Verification items for this drawing (mm, ordinates from the low corner). Give positions to 0.01 mm unless a question says otherwise; leave off trailing zeros. Write each loop counter-clockwise with the first axis right and the second up, starting at its lowest first coordinate (ties: lowest second). Pieces come first, ordered by that corner, then holes. Notation, with made-up numbers: (25, -39) -> (66, -39) arc R26 cw to (66, -20) -> close; hole circle Ø9 at (-7.5, 60). An arc over 180 degrees is marked (long way). Answer as a JSON object with one key per item and string values.
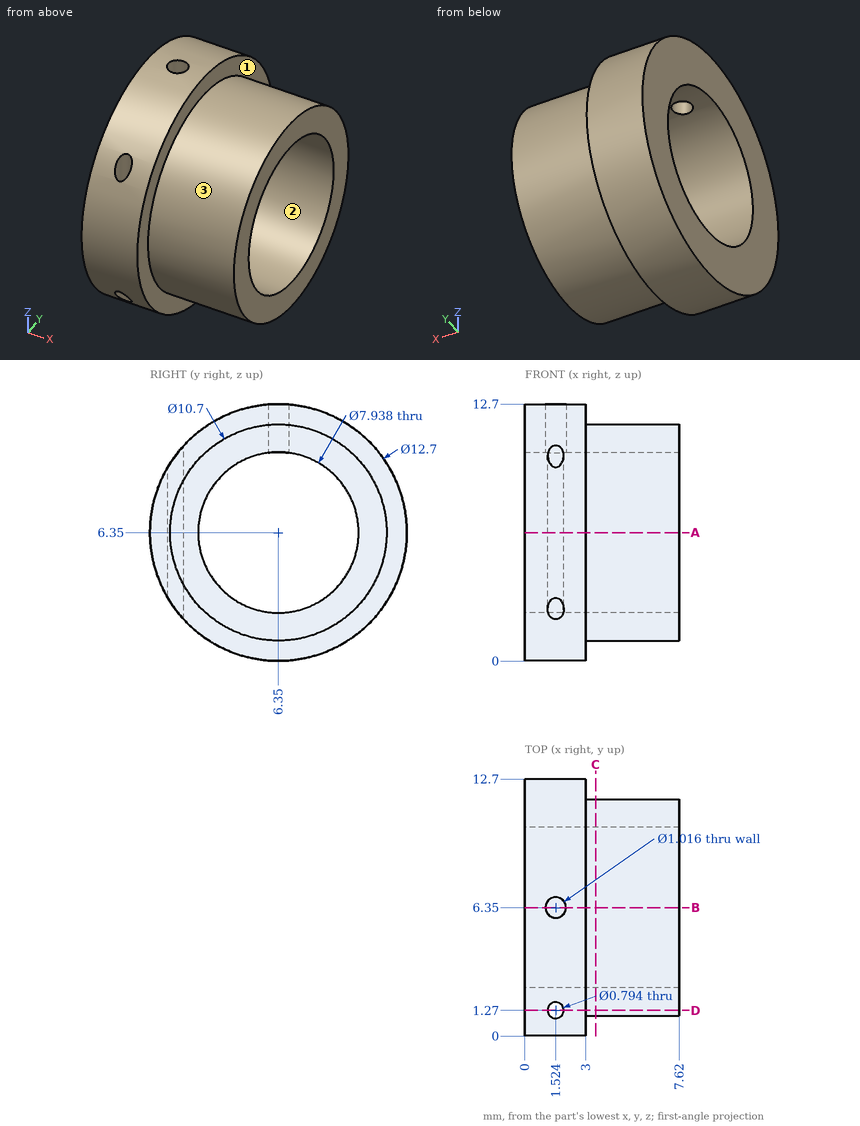
1. Scan lines: L1, parallel to Y at x = 1.5, z = 9 (1 decimal); L2, parallel to Z at x = 6.25, y = 6.5 (1 decimal); L3, parallel to Z at x = 1.75, y = 5.5. Record each from-to range of solid material in increasing order. Write a range as [from, to].
Determined:
{"L1": "[0.6, 0.9], [1.7, 3.4], [9.3, 12.1]", "L2": "[1, 2.4], [10.3, 11.7]", "L3": "[0.06, 2.47], [10.23, 12.64]"}
2. Sectioned sample at D-D, the plane y = 1.27. Enter the section's corners in (x, z).
Determined:
{"outline": "(0, 2.54) -> (1.13, 2.54) -> (1.13, 10.16) -> (0, 10.16) -> close; (1.92, 2.54) -> (3, 2.54) -> (3, 4.67) -> (7.62, 4.67) -> (7.62, 8.03) -> (3, 8.03) -> (3, 10.16) -> (1.92, 10.16) -> close"}
3. Mould release check, pull along Y, two halves, no side actions. Record for the marked faces 1, 2 and 3: released by +Y, released by -Y, zero draft, split by the parting line, or undercut.
Determined:
{"face 1": "zero draft", "face 2": "undercut", "face 3": "split by the parting line"}
4. Go/stop test with flat-tipped pins: P1, Ø2, axis at x = 2.5, z = 7.5, coming from the +Y side; P2, Ø1, axis at y = 7.5, z = 9.5, coming from the -X side; P3, Ø1.5, axis at x = 2, z = 11, coming from the -Y side. Record where each tip stops, or that it passes through.
Determined:
{"P1": "y = 12.7", "P2": "through", "P3": "y = 1.34"}
5. Sectioned sample at C-C, the plane x = 3.5. Enter the section's corners in (y, z).
Determined:
{"outline": "circle Ø10.7 at (6.35, 6.35); hole circle Ø7.94 at (6.35, 6.35)"}
6. Sectioned sample at B-B, the plane y = 6.35. Enter the section's corners in (x, z) (1 decimal).
Determined:
{"outline": "(0, 0) -> (3, 0) -> (3, 1) -> (7.6, 1) -> (7.6, 2.4) -> (0, 2.4) -> close; (0, 10.3) -> (1, 10.3) -> (1, 12.7) -> (0, 12.7) -> close; (2, 10.3) -> (7.6, 10.3) -> (7.6, 11.7) -> (3, 11.7) -> (3, 12.7) -> (2, 12.7) -> close"}
7. Sectioned sample at A-A, the plane z = 6.35. Enter the section's corners in (x, y) (1 decimal).
Determined:
{"outline": "(0, 0) -> (3, 0) -> (3, 1) -> (7.6, 1) -> (7.6, 2.4) -> (0, 2.4) -> close; (0, 10.3) -> (7.6, 10.3) -> (7.6, 11.7) -> (3, 11.7) -> (3, 12.7) -> (0, 12.7) -> close; hole circle Ø0.8 at (1.5, 1.3)"}
